```python
from build123d import *

# Parameters (mm, degrees)
F1_DEPTH       = 30
F2_R           = 5
F3_R           = 5
F6_D           = 10
F6_CBORE_D     = 15
F6_CBORE_DEPTH = 5
F7_D           = 10
F7_CBORE_D     = 15
F7_CBORE_DEPTH = 5
F9_DEPTH       = 9.001


with BuildPart() as f1:
    # F0 (on Front) → F1 (new body)
    with BuildSketch(Plane.XZ):
        Polygon((0, 0), (60, 0), (60, 12), (9, 12), (9, 40), (0, 40), align=None)
    extrude(amount=F1_DEPTH)

    # F2
    f2_edges = [f1.edges().sort_by_distance(p)[0] for p in [
        (4.5, -30, 40),
    ]]
    fillet(f2_edges, radius=F2_R)

    # F3
    f3_edges = [f1.edges().sort_by_distance(p)[0] for p in [
        (4.5, 0, 40),
    ]]
    fillet(f3_edges, radius=F3_R)

    # F6 (through all)
    with Locations(Plane.XY.offset(12)):
        with Locations((44, -15)):
            CounterBoreHole(F6_D / 2, F6_CBORE_D / 2, F6_CBORE_DEPTH)

    # F7 (through all)
    with Locations(Plane.XY.offset(12)):
        with Locations((25, -15)):
            CounterBoreHole(F7_D / 2, F7_CBORE_D / 2, F7_CBORE_DEPTH)

    # F8 (on face) → F9 (cut, through all)
    with BuildSketch(Plane.YZ.offset(9)):
        with BuildLine():
            ThreePointArc((-12, 30), (-15, 33), (-18, 30))
            Line((-18, 30), (-18, 23))
            ThreePointArc((-18, 23), (-15, 20), (-12, 23))
            Line((-12, 23), (-12, 30))
        make_face()
    extrude(amount=-F9_DEPTH, mode=Mode.SUBTRACT)


solid = f1.part
```
Check sheet for the modelled part. Datum: model origin and axes. Units: mm. A direction names the side the tool comes from. Round coordinates to 2 decimals unless told otherwise and drop trailing zeros. Order: outer loops, then holes, each group sorted by start corner. A loop starts at its lowest first (then second) coordinate and runs counter-clockwise, first axis right, second up. Notation, with made-up numbers: (53, 37) -> (68, 37) arc R12 ccw to (68, 42) -> close; hole circle Ø11 at (62.5, -27). An arc over 180 degrees is marked (long way). One line per item, written item: value. Start each with the question number.
Q1. Cross-section at C-C (z = 31.5). Record the boundary of the cut face in (x, y), and give its area (3 significant figures).
Q2. Gauge pin test, flat ends, axial feed: pin 1 Ø13.5 at (x, y) = (25, -15) entering from +Z; pin 2 Ø15 at (x, y) = (25.5, -18.5) entering from +Z; pin 3 Ø6 at (x, y) = (43, -5.5) entering from -Z; pin 4 Ø5 at (y, z) = (-17, 27) entering from +X. Record the tip position at first contact, or that the pin passes through.
Q3. Cross-section at B-B (x = 4). Record the boundary of the cut face in (y, z), and give its area (3 significant figures).
Q4. Cross-section at A-A (y = -15). Record the boundary of the cut face in (x, z), and give its area (3 significant figures).
Q5. Set-up check for faces 1 (the face through (30, -11, 0)), 2 (the face through (5, -18, 27)), 3 (the face through (51.154, -12.747, 9.535)), 4 (the face through (9, -11, 26)): record each of +Z, -Z, +X, -X, +Y, -Y from which the full face is reachable in a straight line by a thin tool's end or side.
Q6. Cross-section at D-D (z = 4). Record the boundary of the cut face in (x, y).
Q7. Thickness scan on line 1 (Y direction, x = 44, z = 9.3); line 2 (X direction, y = -15.25, z = 13.5); line 3 (Z direction, x = 51, y = -12). Record the ranges inside material, lowest first.
Q8. Mould release check, pull along X, two halves, no side actions. Record for faces 5 (the face through (23, -30, 10)), 6 (the face through (0, -18, 20)), 7 (the face through (48, -18, 3)), 8 (the face through (17.507, -14.67, 9.535)): pulls with the +X half, pulls with the -X half, needs draft (parallel to the pull), parting line crosses it, or undercut.
Completed:
1. outline: (0, -30) -> (9, -30) -> (9, -17.6) -> (0, -17.6) -> close; (0, -12.4) -> (9, -12.4) -> (9, 0) -> (0, 0) -> close
1. area: 223 mm²
2. pin 1: stops at z = 7
2. pin 2: stops at z = 12
2. pin 3: stops at z = 0
2. pin 4: stops at x = 9
3. outline: (-30, 0) -> (0, 0) -> (0, 35) arc R5 ccw to (-5, 40) -> (-25, 40) arc R5 ccw to (-30, 35) -> close; hole (-18, 23) arc R3 ccw to (-12, 23) -> (-12, 30) arc R3 ccw to (-18, 30) -> close
3. area: 1,120 mm²
4. outline: (0, 0) -> (20, 0) -> (20, 7) -> (17.5, 7) -> (17.5, 12) -> (9, 12) -> (9, 20) -> (0, 20) -> close; (0, 33) -> (9, 33) -> (9, 40) -> (0, 40) -> close; (30, 0) -> (39, 0) -> (39, 7) -> (36.5, 7) -> (36.5, 12) -> (32.5, 12) -> (32.5, 7) -> (30, 7) -> close; (49, 0) -> (60, 0) -> (60, 12) -> (51.5, 12) -> (51.5, 7) -> (49, 7) -> close
4. area: 565 mm²
5. face 1: -Z, +X, -X, +Y, -Y
5. face 2: +X, -X
5. face 3: +Z
5. face 4: +Z, +X, +Y, -Y
6. outline: (0, -30) -> (60, -30) -> (60, 0) -> (0, 0) -> close; hole circle Ø10 at (25, -15); hole circle Ø10 at (44, -15)
7. line 1: y = -30 to -22.5, -7.5 to 0
7. line 2: x = 0 to 9
7. line 3: z = 0 to 12
8. face 5: needs draft
8. face 6: pulls with the -X half
8. face 7: undercut
8. face 8: undercut
